Build history of the part. All positions in model axes, mm. A direction names the side the tool comes from. Give positions to 0.01 mm unless a question says otherwise; leave off trailing zeros. Loops run counter-clockwise (first coordinate to the right, second up) from the corner with the lowest first, then second, coordinate; pieces in that order, holes last. Notation, with made-up numbers: M 3.5,5.5 L 47.5,5.5 A8 ccw 47.5,13.5 Z; hole C 34.25,23.25 d9. An arc over 180 degrees is marked long. Put each result on its own line as item: value.
```python
from build123d import *

# Parameters (mm, degrees)
SKETCH1_R            = 28
BOSS_EXTRUDE1_DEPTH  = 20
SKETCH2_R            = 27.20625
CUT_EXTRUDE1_DEPTH   = 19.20625
M3_CLEARANCE_HOLE1_D = 3.4
SKETCH5_R            = 2.5
CUT_EXTRUDE2_DEPTH   = 45.362146026


with BuildPart() as part:
    # Sketch1 → Boss-Extrude1 (new body)
    with BuildSketch(Plane(origin=(0, 0, 0), x_dir=(1, 0, 0), z_dir=(0, 1, 0))):
        with Locations(Location((0, 0, 0), (0, 0, 270))):
            Circle(SKETCH1_R)
    extrude(amount=BOSS_EXTRUDE1_DEPTH)

    # Sketch2 → Cut-Extrude1 (cut)
    with BuildSketch(Plane(origin=(0, 20, 0), x_dir=(1, 0, 0), z_dir=(0, 1, 0))):
        with Locations(Location((0, 0, 0), (0, 0, 270))):
            Circle(SKETCH2_R)
    extrude(amount=-CUT_EXTRUDE1_DEPTH, mode=Mode.SUBTRACT)

    # M3 Clearance Hole1 (through all)
    with Locations(Plane(origin=(0, 0, 0), x_dir=(-1, 0, 0), z_dir=(0, -1, 0))):
        with Locations((0, 8), (0, -8), (-8.700000126, 0), (8.700000126, 0)):
            Hole(M3_CLEARANCE_HOLE1_D / 2)

    # Sketch5 → Cut-Extrude2 (cut, through all)
    with BuildSketch(Plane.XZ):
        with Locations(Location((0, 0, 0), (0, 0, 270))):
            Circle(SKETCH5_R)
    extrude(amount=-CUT_EXTRUDE2_DEPTH, mode=Mode.SUBTRACT)


solid = part.part
```
Q1. Drop flat-ended pins along their axis: pin 1 Ø5.5 at (x, z) = (0, -8) entering from +Y; pin 2 Ø1.5 at (x, y) = (-4.5, 14) entering from -Z; pin 3 Ø2.5 at (x, z) = (-8.7, 0) entering from +Y; pin 4 Ø3 at (y, z) = (14.5, -2) entering from +X. Give the stop position or say it passes through.
Here are the results:
pin 1: y = 0.79
pin 2: z = -27.75
pin 3: through
pin 4: x = 28
Q2. Slice it at A-A (z = 0). List the corners of the cut face in (x, y), and give its area (3 significant figures).
Here are the results:
outline: M -28,0 L -10.4,0 L -10.4,0.79 L -27.21,0.79 L -27.21,20 L -28,20 Z; M -7,0 L -2.5,0 L -2.5,0.79 L -7,0.79 Z; M 2.5,0 L 7,0 L 7,0.79 L 2.5,0.79 Z; M 10.4,0 L 28,0 L 28,20 L 27.21,20 L 27.21,0.79 L 10.4,0.79 Z
area: 65.6 mm²
Q3. Slice it at B-B (x = 0). List the corners of the cut face in (y, z).
Here are the results:
outline: M 0,-28 L 20,-28 L 20,-27.21 L 0.79,-27.21 L 0.79,-9.7 L 0,-9.7 Z; M 0,-6.3 L 0.79,-6.3 L 0.79,-2.5 L 0,-2.5 Z; M 0,2.5 L 0.79,2.5 L 0.79,6.3 L 0,6.3 Z; M 0,9.7 L 0.79,9.7 L 0.79,27.21 L 20,27.21 L 20,28 L 0,28 Z
Q4. Slice it at D-D (x = -8.7). List the corners of the cut face in (y, z), and give its area (3 significant figures).
Here are the results:
outline: M 0,-26.61 L 20,-26.61 L 20,-25.78 L 0.79,-25.78 L 0.79,-1.7 L 0,-1.7 Z; M 0,1.7 L 0.79,1.7 L 0.79,25.78 L 20,25.78 L 20,26.61 L 0,26.61 Z
area: 71.7 mm²
Q5. Probe line 1 (Y direction, x = -11, z = 14.5); line 2 (X direction, y = 17, z = -14); line 3 (Z direction, x = -8.7, y = 0.4). List the from-to ranges inside material, lowest first. Write a range as from..to.
Here are the results:
line 1: 0..0.79
line 2: -24.25..-23.33, 23.33..24.25
line 3: -26.61..-1.7, 1.7..26.61
Q6. Slice it at C-C (y = 8.25). List the corners of the cut face in (x, z), and give its area (3 significant figures).
Here are the results:
outline: C 0,0 d56; hole C 0,0 d54.41
area: 138 mm²
Q7. Tool access for faces 4 (the flat face through (0, 0, 6)), 5 (the cylindrical face through (8.17, 10.53, 25.95)): list every direction of +Z, -Z, +X, -X, +Y, -Y with a clear straight run to the whole face (end or side of a thin tool).
Here are the results:
face 4: +Z, -Z, +X, -X, -Y
face 5: +Y
Q8. Mould opens along Z. For faces 1 (the flat face through (23, 20, -15)), 2 (the cylindrical face through (-0.221, 0.402, -9.686)), 3 (the cylindrical face through (-27.334, 9.86, -6.07)) say: pulls with the +Z half, pulls with the -Z half, needs draft (parallel to the pull), parting line crosses it, or undercut.
Here are the results:
face 1: needs draft
face 2: undercut
face 3: parting line crosses it
